from build123d import *

# Parameters (mm, degrees)
SKETCH1_W           = 750
SKETCH1_H           = 50
SKETCH1_R           = 1.25
BOSS_EXTRUDE1_DEPTH = 2
FILLET1_R           = 1
CUT_EXTRUDE1_DEPTH  = 2


with BuildPart() as part:
    # Sketch1 → Boss-Extrude1 (new body)
    with BuildSketch(Plane(origin=(0, 0, 0), x_dir=(1, 0, 0), z_dir=(0, 1, 0))):
        with Locations((375, 25)):
            Rectangle(SKETCH1_W, SKETCH1_H)
        with Locations((10, 42)):
            Circle(SKETCH1_R, mode=Mode.SUBTRACT)
        with Locations((10, 8)):
            Circle(SKETCH1_R, mode=Mode.SUBTRACT)
        with Locations((740, 8)):
            Circle(SKETCH1_R, mode=Mode.SUBTRACT)
        with Locations((740, 42)):
            Circle(SKETCH1_R, mode=Mode.SUBTRACT)
    extrude(amount=BOSS_EXTRUDE1_DEPTH)

    # Fillet1
    fillet1_edges = [part.edges().sort_by_distance(p)[0] for p in [
        (0, 1, -50),
        (750, 1, -50),
        (750, 1, 0),
        (0, 1, 0),
    ]]
    fillet(fillet1_edges, radius=FILLET1_R)

    # Sketch2 → Cut-Extrude1 (cut)
    with BuildSketch(Plane(origin=(0, 2, 0), x_dir=(1, 0, 0), z_dir=(0, 1, 0))):
        with BuildLine():
            Line((741.815018385, 30.48633271), (750, 32.679491924))
            Line((750, 32.679491924), (750, 17.320508076))
            Line((750, 17.320508076), (741.815018385, 19.51366729))
            ThreePointArc((741.815018385, 19.51366729), (740.31863757, 19.450157279), (739.127091147, 18.542739963))
            ThreePointArc((739.127091147, 18.542739963), (718.819660113, 25), (739.127091147, 31.457260037))
            ThreePointArc((739.127091147, 31.457260037), (740.31863757, 30.549842721), (741.815018385, 30.48633271))
        make_face()
        with BuildLine():
            Line((0, 32.679491924), (0, 17.320508076))
            Line((0, 17.320508076), (8.184981615, 19.51366729))
            ThreePointArc((8.184981615, 19.51366729), (9.68136243, 19.450157279), (10.872908853, 18.542739963))
            ThreePointArc((10.872908853, 18.542739963), (31.180339887, 25), (10.872908853, 31.457260037))
            ThreePointArc((10.872908853, 31.457260037), (9.68136243, 30.549842721), (8.184981615, 30.48633271))
            Line((8.184981615, 30.48633271), (0, 32.679491924))
        make_face()
    extrude(amount=-CUT_EXTRUDE1_DEPTH, mode=Mode.SUBTRACT)


solid = part.part
Geometry: final body of the model. Coordinates: model frame, mm. Give positions to 0.01 mm unless a question says otherwise; leave off trailing zeros. Write each loop counter-clockwise with the first axis right and the second up, starting at its lowest first coordinate (ties: lowest second). Pieces come first, ordered by that corner, then holes.
(1) Cut plane B-B, the plane y = 1.55. Return loops of the section in (x, z), then the cut area to 3 significant figures.
(2) Ray query, line 1 (X direction, y = 0.45, z = -8); line 2 (Z direction, x = 20, y = 0.9); line 3 (Z direction, x = 10, y = 1.65). Return the intervals inside material, ascending.
(3) Mould query, pull axis Z, two halves, no side actions, for faces 1 (the cylindrical face through (718.827, 1.014, -24.605)), 2 (the flat face through (370, 0, -25)). Classes: released by +Z, released by -Z, zero draft, split by the parting line, or undercut.
(4) Cut plane A-A, the plane x = 20. Return loops of the section in (y, z), then the cut area to 3 significant figures.
(5) First-contact query: P1, Ø4, axis at x = 740, z = -8, coming from the -Y side. Flat tip, straight axial feed; report the tip coordinate or a pass-through.
Values follow:
1. outline: (0, -49) arc R1 ccw to (1, -50) - (749, -50) arc R1 ccw to (750, -49) - (750, -32.68) - (741.82, -30.49) arc R2.5 ccw to (739.13, -31.46) arc R11.18 cw (long way) to (739.13, -18.54) arc R2.5 ccw to (741.82, -19.51) - (750, -17.32) - (750, -1) arc R1 ccw to (749, 0) - (1, 0) arc R1 ccw to (0, -1) - (0, -17.32) - (8.18, -19.51) arc R2.5 ccw to (10.87, -18.54) arc R11.18 cw (long way) to (10.87, -31.46) arc R2.5 ccw to (8.18, -30.49) - (0, -32.68) - close; hole circle Ø2.5 at (10, -42); hole circle Ø2.5 at (10, -8); hole circle Ø2.5 at (740, -42); hole circle Ø2.5 at (740, -8)
1. area: 36,500 mm2
2. line 1: x = 0 to 8.75, 11.25 to 738.75, 741.25 to 750
2. line 2: z = -50 to -36.18, -13.82 to 0
2. line 3: z = -50 to -43.25, -40.75 to -30.69, -19.31 to -9.25, -6.75 to 0
3. face 1: undercut
3. face 2: zero draft
4. outline: (0, -50) - (2, -50) - (2, -36.18) - (0, -36.18) - close; (0, -13.82) - (2, -13.82) - (2, 0) - (0, 0) - close
4. area: 55.3 mm2
5. P1: stops at y = 0
